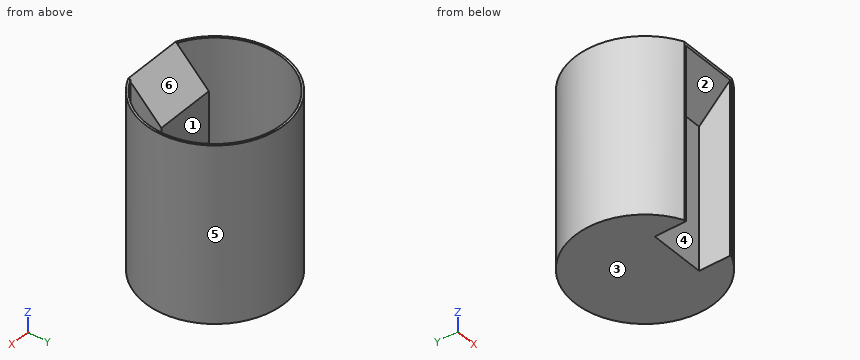
from build123d import *

# Parameters (mm, degrees)
F3_DEPTH = 1.27
F4_DEPTH = 38.1
F7_DEPTH = 1.27
F8_DEPTH = 112.7691580497
F9_DEPTH = 1.27


with BuildPart() as f3:
    # F2 (on plane+point) → F3 (new body)
    with BuildSketch(Plane.YZ.offset(19.05)):
        Polygon((-40.1609262841, 0), (-20.3232679032, 0), (-20.3232679032, 1.27), (-20.3232679032, 91.1354484446), (-38.8909262841, 109.7031068255), (-40.1609262841, 110.9731068255), align=None)
    extrude(amount=-F3_DEPTH)

    # F2 (on plane+point) → F4 (join)
    with BuildSketch(Plane.YZ.offset(19.05)):
        Polygon((-20.3232679032, 0), (-19.0532679032, 0), (-19.0532679032, 91.6614996688), (-40.1609262841, 112.7691580497), (-40.1609262841, 110.9731068255), (-38.8909262841, 109.7031068255), (-20.3232679032, 91.1354484446), (-20.3232679032, 1.27), align=None)
    extrude(amount=-F4_DEPTH)

    # F6 (on offset) → F7 (join)
    with BuildSketch(Plane(origin=(-19.05, 0, 0), x_dir=(0, -1, 0), z_dir=(-1, 0, 0))):
        Polygon((20.3232679032, 0), (40.1597768068, 0), (40.1609262841, 110.9731068255), (20.3232679032, 91.1354484446), align=None)
    extrude(amount=-F7_DEPTH)

    # F0 (on Top) → F8 (join, through all)
    with BuildSketch(Plane.XY):
        with BuildLine():
            Line((19.05, -38.7506116081), (19.05, -40.1609262841))
            ThreePointArc((19.05, -40.1609262841), (0, 44.45), (-19.05, -40.1609262841))
            Line((-19.05, -40.1609262841), (-19.05, -38.7506116081))
            ThreePointArc((-19.05, -38.7506116081), (0, 43.18), (19.05, -38.7506116081))
        make_face()
    extrude(amount=F8_DEPTH)

    # F0 (on Top) → F9 (join)
    with BuildSketch(Plane.XY):
        with BuildLine():
            Line((19.05, -19.0532679032), (19.05, -38.7506116081))
            ThreePointArc((19.05, -38.7506116081), (0, 43.18), (-19.05, -38.7506116081))
            Line((-19.05, -38.7506116081), (-19.05, -19.0532679032))
            Line((-19.05, -19.0532679032), (0, -19.0532679032))
            Line((0, -19.0532679032), (19.05, -19.0532679032))
        make_face()
    extrude(amount=F9_DEPTH)


solid = f3.part
Read the model definition and answer for the solid it produces. Units are mm, in the model's axes. Face numbers are marked on the shaded views. A direction names the side the tool comes from. Round coordinates to 2 decimals unless told otherwise and drop trailing zeros. Loops run counter-clockwise (first coordinate to the right, second up) from the corner with the lowest first, then second, coordinate; pieces in that order, holes last.
Q1. Section C-C on y = 0 is taken. Write down the section's boundary in (x, z).
Q2. Section A-A on x = 0 is taken. Write down the section's boundary in (y, z), and give its area (3 significant figures).
Q3. Which of the six approach directions +Z, -Z, +X, -X, +Y, -Y give full straight-line access (tool end or side, diameter ignored) to the marked faces 1 and 2?
Q4. Consider probe 1 along X at (y, z) = (0, 68.5); probe 2 along Z at (x, y) = (-39, 2.5); probe 3 along X at (y, z) = (-33.5, 34). Determine where each line is inside the solid, lowest interval first.
Q5. Each of these flat-tipped pins is pushed along its axis until it touches: pin 1 (12 mm diameter, centred on y = 21, z = 88.5, fed in from -X); pin 2 (1.5 mm diameter, centred on x = -21.5, y = 0.5, fed in from +Z); pin 3 (0.7 mm diameter, centred on y = -39.5, z = 112.5, fed in from -X). Where does it stop, or does it pass through?
Q6. Determine the mould class of the marked faces 3, 4, 5 and 6 for opening direction Y: released by +Y, released by -Y, zero draft, split by the parting line, or undercut.
Output:
1. outline: (-44.45, 0) - (44.45, 0) - (44.45, 112.77) - (43.18, 112.77) - (43.18, 1.27) - (-43.18, 1.27) - (-43.18, 112.77) - (-44.45, 112.77) - close
2. outline: (-40.16, 110.97) - (-20.32, 91.14) - (-20.32, 0) - (44.45, 0) - (44.45, 112.77) - (43.18, 112.77) - (43.18, 1.27) - (-19.05, 1.27) - (-19.05, 91.66) - (-40.16, 112.77) - close
2. area: 375 mm2
3. face 1: +Z
3. face 2: -Z, -Y
4. probe 1: x = -44.45 to -43.18, 43.18 to 44.45
4. probe 2: z = 0 to 1.27
4. probe 3: x = -29.22 to -27.24, -19.05 to -17.78, 17.78 to 19.05, 27.24 to 29.22
5. pin 1: stops at x = -41.84
5. pin 2: stops at z = 1.27
5. pin 3: stops at x = -21.05
6. face 3: zero draft
6. face 4: released by -Y
6. face 5: split by the parting line
6. face 6: undercut
